Could you check a few things on this model? Use its own coordinates, in mm. Face numbers are marked on the shaded views. A direction names the side the tool comes from. Coordinates: 2 decimals unless noted, no trailing zeros. One line per question, with ' | ' between items. Start each with the question number.
1. I'm going to push flat-ended pins straight in: P1, Ø2, axis at y = 33.5, z = 13, coming from the -X side; P2, Ø5.5, axis at x = 142.21, y = 111.19, coming from the +Z side; P3, Ø4, axis at x = 149.14, y = 107.19, coming from the -Z side; P4, Ø18.5, axis at x = 81.5, y = 26, coming from the +Z side. Where does each tip first touch, or does it pass through?
2. Please list where these lines run through material, in increasing order: L1, parallel to X at y = 81.5, z = 22; L2, parallel to X at y = 82, z = 30.5; L3, parallel to X at y = 78, z = 29. Write a range as [from, to].
3. Which directions (+Z, -Z, +X, -X, +Y, -Y) give clear straight access to the entire face, cutting with the end or side of a thin tool? Please do the marked faces 5, 6 and 7.
4. We'd pull the mould along X, two halves only. Please class the marked faces 1, 2, 3 and 4: pulls with the +X half, pulls with the -X half, needs draft (parallel to the pull), parting line crosses it, or undercut.
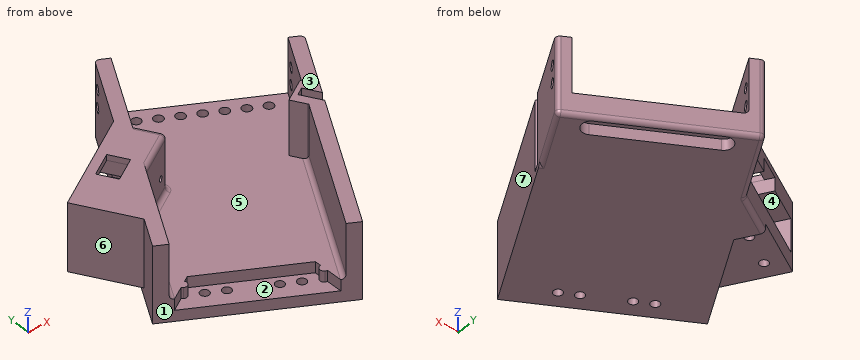
from build123d import *

# Parameters (mm, degrees)
SKETCH_2_W               = 109.92
SKETCH_2_H               = 76
EXTRUDE_1_DEPTH          = 10
CUT_EXTRUDE_1_DEPTH      = 5
SKETCH_4_R               = 2
CUT_EXTRUDE_2_DEPTH      = 92.808295873
SKETCH_5_W               = 109.92
SKETCH_5_H               = 6
EXTRUDE_2_DEPTH          = 25
CUT_EXTRUDE_3_DEPTH      = 104.340627651
CUT_EXTRUDE_3_DEPTH_BACK = 104.340627651
SKETCH_7_R               = 2.1
SKETCH_9_R               = 2.1
CUT_EXTRUDE_4_DEPTH      = 96.019804204
CUT_EXTRUDE_5_DEPTH      = 5
EXTRUDE_3_DEPTH          = 35
EXTRUDE_4_DEPTH          = 35
SKETCH_13_W              = 46
SKETCH_13_H              = 15
SKETCH_13_W_2            = 12
SKETCH_13_H_2            = 6
CUT_EXTRUDE_6_DEPTH      = 15
CUT_EXTRUDE_7_DEPTH      = 15
SKETCH_15_R              = 1.25
CUT_EXTRUDE_8_DEPTH      = 28.709519
EXTRUDE_5_DEPTH          = 35
CUT_EXTRUDE_10_DEPTH     = 4
CUT_EXTRUDE_11_REACH     = 116.42
SKETCH_22_R              = 2
CUT_EXTRUDE_12_DEPTH     = 3.5
CUT_EXTRUDE_14_REACH     = 117.568
EXTRUDE_6_DEPTH          = 3
EXTRUDE_7_REACH          = 117.568
SKETCH_27_W              = 4.526779154
SKETCH_27_H              = 4.806116501
FILLET_1_R               = 2
CUT_EXTRUDE_15_REACH     = 117.568
SKETCH_28_W              = 4.526779154
SKETCH_28_H              = 4.806116501


with BuildPart() as part:
    # 草圖2 → 填料-伸長1 (new body)
    with BuildSketch(Plane.XY):
        with Locations((12.52544527, 24.044160626)):
            Rectangle(SKETCH_2_W, SKETCH_2_H)
    extrude(amount=EXTRUDE_1_DEPTH)

    # 草圖3 → 除料-伸長1 (cut)
    with BuildSketch(Plane.XY.offset(10)):
        with BuildLine():
            Line((67.48544527, -6.055839374), (67.48544527, 54.144160626))
            Line((67.48544527, 54.144160626), (61.24181631, 50.538464901))
            ThreePointArc((61.24181631, 50.538464901), (61.408690367, 50.105080914), (61.46544527, 49.644160626))
            ThreePointArc((61.46544527, 49.644160626), (60.088104264, 47.81746208), (57.95299519, 48.639170705))
            Line((57.95299519, 48.639170705), (55.48544527, 47.214160626))
            Line((55.48544527, 47.214160626), (55.48544527, 0.874160626))
            Line((55.48544527, 0.874160626), (57.95299519, -0.550849453))
            ThreePointArc((57.95299519, -0.550849453), (60.088104264, 0.270859171), (61.46544527, -1.555839374))
            ThreePointArc((61.46544527, -1.555839374), (61.408690367, -2.016759663), (61.24181631, -2.45014365))
            Line((61.24181631, -2.45014365), (67.48544527, -6.055839374))
        make_face()
    extrude(amount=-CUT_EXTRUDE_1_DEPTH, mode=Mode.SUBTRACT)

    # 草圖4 → 除料-伸長2 (cut, through all)
    with BuildSketch(Plane.XY.offset(5)):
        with Locations((59.56544527, 41.644160626)):
            Circle(SKETCH_4_R)
        with Locations((59.56544527, 33.644160626)):
            Circle(SKETCH_4_R)
        with Locations((59.56544527, 6.444160626)):
            Circle(SKETCH_4_R)
        with Locations((59.56544527, 14.444160626)):
            Circle(SKETCH_4_R)
    extrude(amount=-CUT_EXTRUDE_2_DEPTH, mode=Mode.SUBTRACT)

    # 草圖5 → 填料-伸長2 (add)
    with BuildSketch(Plane.XY.offset(10)):
        with Locations((12.52544527, -10.955839374)):
            Rectangle(SKETCH_5_W, SKETCH_5_H)
        with Locations((12.52544527, 59.044160626)):
            Rectangle(SKETCH_5_W, SKETCH_5_H)
    extrude(amount=EXTRUDE_2_DEPTH)

    # 草圖7 → 除料-伸長3 (cut, two sides: drawn at the far end of the back side and taken through both)
    with BuildSketch(Plane(origin=(0, -7.955839374, 0), x_dir=(1, 0, 0), z_dir=(0, 1, 0)).offset(-CUT_EXTRUDE_3_DEPTH_BACK)):
        with Locations(Location((-36.43455473, -18, 0), (0, 0, 270))):
            Circle(SKETCH_7_R)
        with Locations(Location((-36.43455473, -26, 0), (0, 0, 270))):
            Circle(SKETCH_7_R)
    extrude(amount=CUT_EXTRUDE_3_DEPTH + CUT_EXTRUDE_3_DEPTH_BACK, mode=Mode.SUBTRACT)

    # 草圖9 → 除料-伸長4 (cut, through all)
    with BuildSketch(Plane.XY.offset(10)):
        with Locations((-36.43455473, 0.044160626)):
            Circle(SKETCH_9_R)
        with Locations((-36.43455473, 8.044160626)):
            Circle(SKETCH_9_R)
        with Locations((-36.43455473, 16.044160626)):
            Circle(SKETCH_9_R)
        with Locations((-36.43455473, 24.044160626)):
            Circle(SKETCH_9_R)
        with Locations((-36.43455473, 32.044160626)):
            Circle(SKETCH_9_R)
        with Locations((-36.43455473, 40.044160626)):
            Circle(SKETCH_9_R)
        with Locations((-36.43455473, 48.044160626)):
            Circle(SKETCH_9_R)
    extrude(amount=-CUT_EXTRUDE_4_DEPTH, mode=Mode.SUBTRACT)

    # 草圖10 → 除料-伸長5 (cut)
    with BuildSketch(Plane(origin=(0, 0, 0), x_dir=(-1, 0, 0), z_dir=(0, 0, -1))):
        with BuildLine():
            Line((32.43455473, 0.044160626), (32.43455473, 48.044160626))
            ThreePointArc((32.43455473, 48.044160626), (36.43455473, 52.044160626), (40.43455473, 48.044160626))
            Line((40.43455473, 48.044160626), (40.43455473, 0.044160626))
            ThreePointArc((40.43455473, 0.044160626), (36.43455473, -3.955839374), (32.43455473, 0.044160626))
        make_face()
    extrude(amount=-CUT_EXTRUDE_5_DEPTH, mode=Mode.SUBTRACT)

    # 草圖11 → 填料-伸長3 (add, through all)
    with BuildSketch(Plane.XY.offset(35)):
        Polygon((51.48544527, 62.044160626), (37.05168854, 87.044160626), (-6.249581649, 62.044160626), align=None)
    extrude(amount=-EXTRUDE_3_DEPTH)

    # 草圖12 → 填料-伸長4 (add)
    with BuildSketch(Plane.XY.offset(35)):
        Polygon((-6.249581649, 62.044160626), (37.05168854, 87.044160626), (47.05168854, 69.72365255), (3.750418351, 44.72365255), align=None)
    extrude(amount=-EXTRUDE_4_DEPTH)

    # 草圖13 → 除料-伸長6 (cut)
    with BuildSketch(Plane(origin=(-28.428305041, 49.239268705, 0), x_dir=(0.8660254037844416, 0.4999999999999949, 0), z_dir=(-0.4999999999999949, 0.8660254037844416, 0))):
        with Locations((50.609783842, -18.9)):
            Rectangle(SKETCH_13_W, SKETCH_13_H)
        with Locations((50.609783842, -29.4)):
            Rectangle(SKETCH_13_W_2, SKETCH_13_H_2)
    extrude(amount=-CUT_EXTRUDE_6_DEPTH, mode=Mode.SUBTRACT)

    # 草圖14 → 除料-伸長7 (cut)
    with BuildSketch(Plane(origin=(0, 0, 32.4), x_dir=(-1, 0, 0), z_dir=(0, 0, -1))):
        Polygon((-22.597205868, 74.080059011), (-27.097205868, 66.285830377), (-16.704901023, 60.285830377), (-12.204901023, 68.080059011), align=None)
    extrude(amount=-CUT_EXTRUDE_7_DEPTH, mode=Mode.SUBTRACT)

    # 草圖15 → 除料-伸長8 (cut)
    with BuildSketch(Plane(origin=(-20.928305041, 36.248887648, 0), x_dir=(0.8660254037844417, 0.4999999999999947, 0), z_dir=(-0.49999999999999484, 0.8660254037844418, 0))):
        with Locations(Location((69.109783842, -18.9, 0), (0, 0, 180))):
            Circle(SKETCH_15_R)
        with Locations(Location((32.109783842, -18.9, 0), (0, 0, 180))):
            Circle(SKETCH_15_R)
    extrude(amount=-CUT_EXTRUDE_8_DEPTH, mode=Mode.SUBTRACT)

    # 草圖18 → 填料-伸長5 (add)
    with BuildSketch(Plane.XY.offset(35)):
        Polygon((-13.593592417, -13.522826672), (-13.343592417, -13.955839374), (-8.724790263, -13.955839374), (-10.129490801, -11.522826672), align=None)
        Polygon((-17.093592417, -7.460648846), (-13.593592417, -13.522826672), (-10.129490801, -11.522826672), (-6.665389186, -9.522826672), (-3.201287571, -7.522826672), (-6.701287571, -1.460648846), align=None)
        Polygon((-3.201287571, -7.522826672), (-6.665389186, -9.522826672), (-4.10598811, -13.955839374), (0.512814044, -13.955839374), align=None)
    extrude(amount=-EXTRUDE_5_DEPTH)

    # 草圖21 → 除料-伸長10 (cut)
    with BuildSketch(Plane(origin=(0, 0, 0), x_dir=(-1, 0, 0), z_dir=(0, 0, -1))):
        Polygon((-37.05168854, 87.044160626), (-43.05168854, 76.65185578), (-51.48544527, 62.044160626), (-17.750418351, 62.044160626), (-11.750418351, 72.436465471), align=None)
    extrude(amount=-CUT_EXTRUDE_10_DEPTH, mode=Mode.SUBTRACT)

    # 草圖22 → 除料-伸長11 (cut, up to next)
    with BuildSketch(Plane(origin=(0, 0, 4), x_dir=(-1, 0, 0), z_dir=(0, 0, -1)), mode=Mode.PRIVATE) as cut_extrude_11_sk1:
        with Locations((-34.12348531, 76.115957396)):
            Circle(SKETCH_22_R)
    cut_extrude_11_tool1 = extrude(cut_extrude_11_sk1.sketch, amount=-CUT_EXTRUDE_11_REACH, mode=Mode.PRIVATE) & part.part
    # 草圖22 → 除料-伸長11 (cut, up to next)
    with BuildSketch(Plane(origin=(0, 0, 4), x_dir=(-1, 0, 0), z_dir=(0, 0, -1)), mode=Mode.PRIVATE) as cut_extrude_11_sk2:
        with Locations((-20.267078849, 68.115957396)):
            Circle(SKETCH_22_R)
    cut_extrude_11_tool2 = extrude(cut_extrude_11_sk2.sketch, amount=-CUT_EXTRUDE_11_REACH, mode=Mode.PRIVATE) & part.part
    add(cut_extrude_11_tool1.solids().sort_by_distance((34.123485, 76.115957, 4))[0], mode=Mode.SUBTRACT)
    add(cut_extrude_11_tool2.solids().sort_by_distance((20.267079, 68.115957, 4))[0], mode=Mode.SUBTRACT)

    # 草圖23 → 除料-伸長12 (cut)
    with BuildSketch(Plane.XY.offset(11.4)):
        Polygon((16.539589727, 69.567103439), (17.14660495, 65.613430145), (20.874094073, 64.162284101), (23.994567972, 66.664811352), (23.387552749, 70.618484646), (19.660063626, 72.06963069), align=None)
        Polygon((30.395996187, 77.567103439), (31.00301141, 73.613430145), (34.730500533, 72.162284101), (37.850974433, 74.664811352), (37.24395921, 78.618484646), (33.516470087, 80.06963069), align=None)
    extrude(amount=-CUT_EXTRUDE_12_DEPTH, mode=Mode.SUBTRACT)

    # 草圖24 → 除料-伸長14 (cut, up to next)
    with BuildSketch(Plane.XY.offset(35), mode=Mode.PRIVATE) as cut_extrude_14_sk1:
        Polygon((-7.570089725, -15.955839374), (-4.10598811, -13.955839374), (-9.165389186, -5.192699653), (-12.629490801, -7.192699653), align=None)
    cut_extrude_14_tool1 = extrude(cut_extrude_14_sk1.sketch, amount=-CUT_EXTRUDE_14_REACH, mode=Mode.PRIVATE) & part.part
    add(cut_extrude_14_tool1.solids().sort_by_distance((-8.367739, -10.57427, 35))[0], mode=Mode.SUBTRACT)

    # 草圖25 → 填料-伸長6 (add)
    with BuildSketch(Plane(origin=(0, 0, 0), x_dir=(-1, 0, 0), z_dir=(0, 0, -1))):
        Polygon((8.724790263, -13.955839374), (4.10598811, -13.955839374), (9.165389186, -5.192699653), (12.629490801, -7.192699653), align=None)
    extrude(amount=-EXTRUDE_6_DEPTH)

    # 填料-伸長7: up to this face of the body (flat: up to its plane)
    extrude_7_end = Plane(part.part.faces().sort_by_distance((14.81484306, 24.690999313, 0))[0])
    # 草圖27 → 填料-伸長7 (add, up to the picked face)
    with BuildSketch(Plane.XY.offset(35), mode=Mode.PRIVATE) as extrude_7_sk1:
        with Locations((-9.842598533, -16.358897625)):
            Rectangle(SKETCH_27_W, SKETCH_27_H)
    extrude_7_tool1 = split(extrude(extrude_7_sk1.sketch, amount=-EXTRUDE_7_REACH, mode=Mode.PRIVATE), bisect_by=extrude_7_end, keep=Keep.BOTH, mode=Mode.PRIVATE)
    add(extrude_7_tool1.solids().sort_by(Axis((-9.842599, -16.358898, 35), (0, 0, -1)))[0])

    # 圓角1
    fillet_1_edges = [part.edges().sort_by_distance(p)[0] for p in [
        (-24.34206819, 62.044160626, 0),
        (-6.249581649, 62.044160626, 17.5),
        (45.421779388, 56.044160626, 10),
        (0.482469159, 50.383906588, 10),
        (13.554265928, 50.383906588, 10),
        (3.750418351, 44.72365255, 22.5),
        (0.482469159, 50.383906588, 35),
        (13.554265928, 50.383906588, 35),
        (2.750418351, 67.240313048, 0),
        (-12.10598811, -16.358897625, 0),
        (-27.27027142, -13.955839374, 0),
        (32.267078849, -7.955839374, 10),
        (-42.43455473, 24.044160626, 0),
        (-22.610017382, 56.044160626, 10),
        (-42.43455473, 62.044160626, 17.5),
        (-42.43455473, -13.955839374, 17.5),
    ]]
    fillet(fillet_1_edges, radius=FILLET_1_R - 0.0001)  # a hair under: the kernel refuses the full size

    # 草圖28 → 除料-伸長15 (cut, up to next)
    with BuildSketch(Plane.XY.offset(35), mode=Mode.PRIVATE) as cut_extrude_15_sk1:
        with Locations((-9.842598533, -16.358897625)):
            Rectangle(SKETCH_28_W, SKETCH_28_H)
    cut_extrude_15_tool1 = extrude(cut_extrude_15_sk1.sketch, amount=-CUT_EXTRUDE_15_REACH, mode=Mode.PRIVATE) & part.part
    add(cut_extrude_15_tool1.solids().sort_by_distance((-9.842599, -16.358898, 35))[0], mode=Mode.SUBTRACT)


with BuildPart() as body_2:
    # 鏡射1: mirrored copy
    add(part.part.mirror(Plane(origin=(51.48544527, 62.044160626, 0), x_dir=(0, 0, 1), z_dir=(0.8660254037844434, 0.4999999999999917, 0))))


solid = body_2.part
Results are:
1) P1: stops at x = 115.26 | P2: stops at z = 10 | P3: passes through | P4: stops at z = 5
2) L1: x = [40.25, 42.56], [57.45, 69.65], [136.99, 140.99], [144.34, 150.48] | L2: x = [39.96, 69.94], [137.86, 141.86], [144.05, 150.76] | L3: x = [42.27, 67.63], [137.12, 141.74], [146.36, 148.45]
3) face 5: +Z | face 6: +Z, -Z, -X | face 7: +Z, -Z, +X, -Y
4) face 1: pulls with the -X half | face 2: undercut | face 3: needs draft | face 4: undercut
